```python
from build123d import *

# Parameters (mm, degrees)
F0_W     = 82.55
F0_H     = 12.7
F1_DEPTH = 190.5
F2_R     = 20.6375
F4_DEPTH = 25.4
F5_W     = 82.55
F5_H     = 25.4
F7_DEPTH = 114.3


with BuildPart() as f1:
    # F0 (on Front) → F1 (new body)
    with BuildSketch(Plane.XZ):
        with Locations((41.275, 6.35)):
            Rectangle(F0_W, F0_H)
    extrude(amount=F1_DEPTH)

    # F2 (on face) → F4 (cut)
    with BuildSketch(Plane(origin=(0, 0, 0), x_dir=(1, 0, 0), z_dir=(0, 0, -1))):
        with Locations((41.275, 76.2)):
            Circle(F2_R)
        with Locations((41.275, 152.4)):
            Circle(F2_R)
    extrude(amount=-F4_DEPTH, mode=Mode.SUBTRACT)

    # F5 (on face) → F7 (join)
    with BuildSketch(Plane.XY.offset(12.7)):
        with Locations((41.275, -12.7)):
            Rectangle(F5_W, F5_H)
    extrude(amount=F7_DEPTH)


solid = f1.part
```
The listing builds one solid part. Answer for the finished solid, in the listing's coordinates (mm). A direction names the side the tool comes from. Give positions to 0.01 mm unless a question says otherwise; leave off trailing zeros. Order: outer loops, then holes, each group sorted by start corner. A loop starts at its lowest first (then second) coordinate and runs counter-clockwise, first axis right, second up. Notation, with made-up numbers: (75, -19.5) -> (88, -19.5) arc R18 cw to (88, 15.5) -> close; hole circle Ø6 at (33, 25.25). An arc over 180 degrees is marked (long way). Answer as CSV lines item,"result". Start each with the question number.
Q1. Find the intervals of material crossed by L1, parallel to X at y = -76.2, z = 5.75; L2, parallel to Y at x = 42, z = 99.5; L3, parallel to Z at x = 20.5, y = -107.5, in increasing order.
Q2. A cutting plane is placed at D-D (x = 72.5). Determine the outline of the cut face in (y, z), then the cut area to 3 significant figures.
Q3. Which of the six approach directions +Z, -Z, +X, -X, +Y, -Y give full straight-line access (tool end or side, diameter ignored) to faces 1 (the flat face through (41, -25.4, 69)), 2 (the flat face through (82.55, -25, 40))?
Q4. Given pin 1 (12 mm diameter, centred on x = 64.5, z = 38.5, fed in from +Y); pin 2 (12 mm diameter, centred on x = 60, z = 51, fed in from -Y); pin 3 (10 mm diameter, centred on x = 46, y = -97.5, fed in from +Z), each flat-ended and moving along its own axis, determine where each tip first touches the part or whether it passes through.
Q5. A cutting plane is placed at B-B (z = 10.5). Count the separate pieces of the cut face and the enclosed holes in it, then the cut area to 3 significant figures.
Q6. A cutting plane is placed at A-A (y = -76.2). Determine the outline of the cut face in (x, z), then the cut area to 3 significant figures.
Q7. A cutting plane is placed at C-C (x = 53.5). Determine the outline of the cut face in (y, z).
Q8. Determine the mould class of faces 3 (the cylindrical face through (36.801, -132.253, 6.261)), 4 (the flat face through (0, -25, 40)), 5 (the flat face through (41, -190.5, 6)) for opening direction Y: pulls with the +Y half, pulls with the -Y half, needs draft (parallel to the pull), parting line crosses it, or undercut.
Results found:
1,L1,"0 to 20.64, 61.91 to 82.55"
1,L2,"-25.4 to 0"
1,L3,"0 to 12.7"
2,outline,"(-190.5, 0) -> (0, 0) -> (0, 127) -> (-25.4, 127) -> (-25.4, 12.7) -> (-190.5, 12.7) -> close"
2,area,"5,320 mm2"
3,face 1,"+Z, +X, -X, -Y"
3,face 2,"+Z, -Z, +X, +Y, -Y"
4,pin 1,"y = 0"
4,pin 2,"y = -25.4"
4,pin 3,"z = 12.7"
5,separate pieces,"1"
5,enclosed holes,"2"
5,area,"13,000 mm2"
6,outline,"(0, 0) -> (20.64, 0) -> (20.64, 12.7) -> (0, 12.7) -> close; (61.91, 0) -> (82.55, 0) -> (82.55, 12.7) -> (61.91, 12.7) -> close"
6,area,"524 mm2"
7,outline,"(-190.5, 0) -> (-169.03, 0) -> (-169.03, 12.7) -> (-190.5, 12.7) -> close; (-135.77, 0) -> (-92.83, 0) -> (-92.83, 12.7) -> (-135.77, 12.7) -> close; (-59.57, 0) -> (0, 0) -> (0, 127) -> (-25.4, 127) -> (-25.4, 12.7) -> (-59.57, 12.7) -> close"
8,face 3,"undercut"
8,face 4,"needs draft"
8,face 5,"pulls with the -Y half"
